```python
from build123d import *

# Parameters (mm, degrees)
BOSS_EXTRUDE1_DEPTH = 15
BOSS_EXTRUDE2_DEPTH = 150
FILLET1_R           = 1
SKETCH3_R           = 35
CUT_EXTRUDE1_DEPTH  = 5


with BuildPart() as part:
    # Sketch1 → Boss-Extrude1 (new body)
    with BuildSketch(Plane(origin=(0, 0, 0), x_dir=(1, 0, 0), z_dir=(0, 1, 0))):
        Polygon((-56.565, 46.565), (-46.565, 56.565), (46.565, 56.565), (56.565, 46.565), (56.565, -46.565), (46.565, -56.565), (-46.565, -56.565), (-56.565, -46.565), align=None)
    extrude(amount=BOSS_EXTRUDE1_DEPTH)

    # Sketch2 → Boss-Extrude2 (add)
    with BuildSketch(Plane(origin=(0, 15, 0), x_dir=(1, 0, 0), z_dir=(0, 1, 0))):
        Polygon((36.565, 46.565), (36.565, 41.565), (41.565, 36.565), (46.565, 36.565), (46.565, -36.565), (41.565, -36.565), (36.565, -41.565), (36.565, -46.565), (-36.565, -46.565), (-36.565, -41.565), (-41.565, -36.565), (-46.565, -36.565), (-46.565, 36.565), (-41.565, 36.565), (-36.565, 41.565), (-36.565, 46.565), align=None)
    extrude(amount=BOSS_EXTRUDE2_DEPTH)

    # Fillet1
    fillet1_edges = [part.edges().sort_by_distance(p)[0] for p in [
        (36.565, 90, -46.565),
        (-36.565, 90, -46.565),
        (-36.565, 90, -41.565),
        (-41.565, 90, -36.565),
        (-46.565, 90, -36.565),
        (-46.565, 90, 36.565),
        (-41.565, 90, 36.565),
        (-36.565, 90, 41.565),
        (-36.565, 90, 46.565),
        (36.565, 90, 46.565),
        (36.565, 90, 41.565),
        (41.565, 90, 36.565),
        (46.565, 90, 36.565),
        (46.565, 90, -36.565),
        (41.565, 90, -36.565),
        (36.565, 90, -41.565),
    ]]
    fillet(fillet1_edges, radius=FILLET1_R)

    # Sketch3 → Cut-Extrude1 (cut)
    with BuildSketch(Plane(origin=(0, 165, 0), x_dir=(1, 0, 0), z_dir=(0, 1, 0))):
        Circle(SKETCH3_R)
    extrude(amount=-CUT_EXTRUDE1_DEPTH, mode=Mode.SUBTRACT)


solid = part.part
```
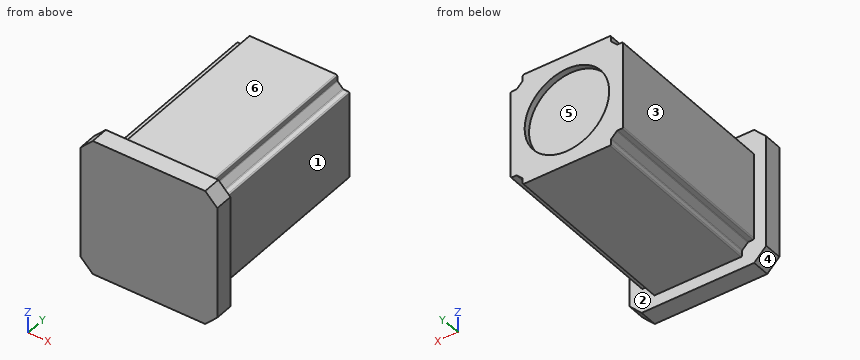
Build history of the part. All positions in model axes, mm. Face numbers are marked on the shaded views. A direction names the side the tool comes from. Give positions to 0.01 mm unless a question says otherwise; leave off trailing zeros. Loops run counter-clockwise (first coordinate to the right, second up) from the corner with the lowest first, then second, coordinate; pieces in that order, holes last.
Item 1: Flat gauge pins, fed straight in: pin 1 (1.1 mm diameter, centred on x = -43, y = 100.5, fed in from -Z) (3 decimals); pin 2 (10 mm diameter, centred on y = 110.5, z = -5, fed in from -X) (3 decimals); pin 3 (3 mm diameter, centred on x = -44, y = 68.5, fed in from +Z) (3 decimals); pin 4 (2 mm diameter, centred on x = 41.5, z = 41.5, fed in from -Y). Where does each tip first touch, or does it go through?
Answers follow:
pin 1: stops at z = -36.565
pin 2: stops at x = -46.565
pin 3: stops at z = 36.565
pin 4: stops at y = 0
Item 2: Slice it at C-C, the plane x = 0. List the corners of the cut face in (y, z) (3 decimals).
Answers follow:
outline: (0, -56.565) - (15, -56.565) - (15, -46.565) - (165, -46.565) - (165, -35) - (160, -35) - (160, 35) - (165, 35) - (165, 46.565) - (15, 46.565) - (15, 56.565) - (0, 56.565) - close
Item 3: Slice it at B-B, the plane z = 0. List the corners of the cut face in (x, y) (3 decimals).
Answers follow:
outline: (-56.565, 0) - (56.565, 0) - (56.565, 15) - (46.565, 15) - (46.565, 165) - (35, 165) - (35, 160) - (-35, 160) - (-35, 165) - (-46.565, 165) - (-46.565, 15) - (-56.565, 15) - close
Item 4: Pull direction Z, two halves, no side cores. Call the marked faces 4, 5 and 6: released by +Z, released by -Z, zero draft, split by the parting line, or undercut.
Answers follow:
face 4: released by -Z
face 5: undercut
face 6: released by +Z
Item 5: Which spindle directions (+Z, -Z, +X, -X, +Y, -Y) get a long thin tool onto all of the face, cutting with end or side? Do the marked faces 1, 2 and 3. Say none if no direction does.
Answers follow:
face 1: +Z, -Z, +X, +Y
face 2: +Y
face 3: +Z, -Z, -X, +Y
Item 6: Drill centre lines: line 1 (Z direction, x = 0, y = 162) (3 decimals); line 2 (Z direction, x = -22, y = 78) (3 decimals). Where is each one in solid material? Low to high.
Answers follow:
line 1: z = -46.565 to -35, 35 to 46.565
line 2: z = -46.565 to 46.565
